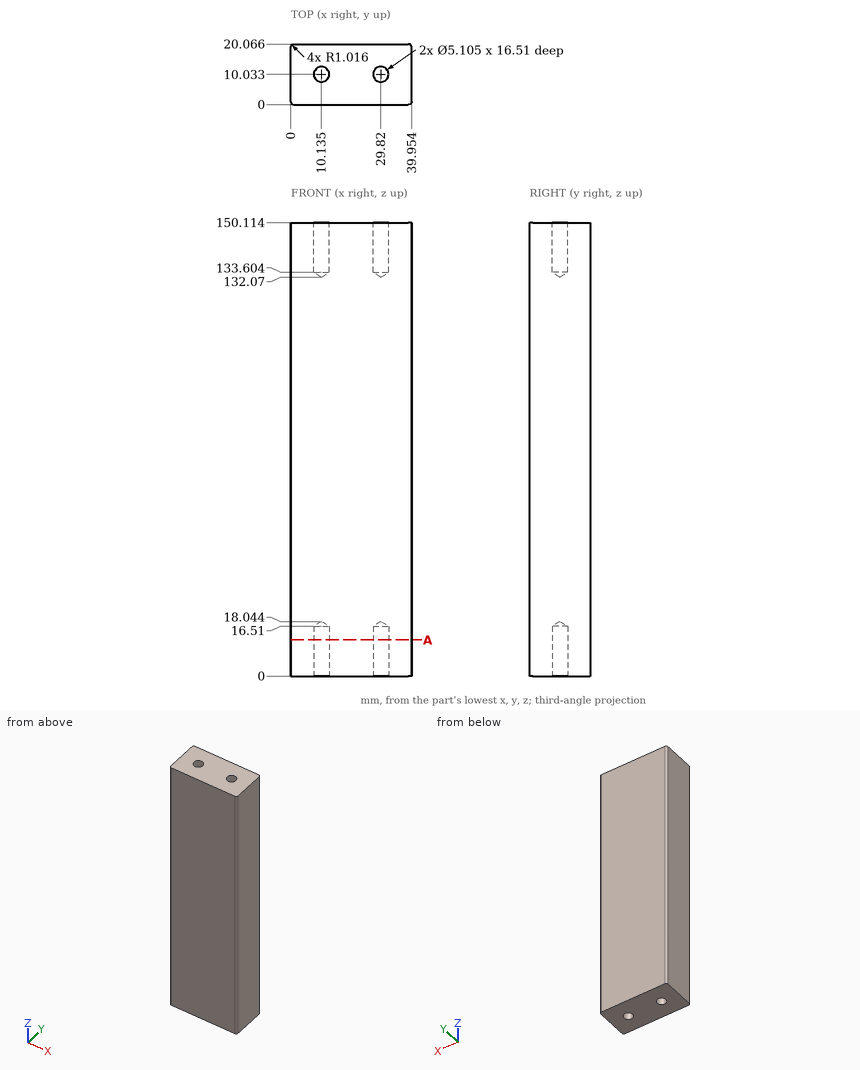
Could you check a few things on this drawing? It's one solid part, dimensions in mm from its lowest x, y, z. Give positions to 0.01 mm unless a question says otherwise; leave off trailing zeros. One line per item, written item: value. Start each with the question number.
1. For P1, Ø8, axis at x = 10.13, y = 10.03, coming from the -Z side; P2, Ø4.5, axis at x = 29.82, y = 10.03, coming from the +Z side (1 decimal); P3, Ø4.5, axis at x = 29.82, y = 10.03, coming from the -Z side, each with a flat end and sliding along its axis, tell me the tip position at first contact or that it passes through.
2. Imagine slicing it at A-A on z = 12. Give the number of separate pieces and of enclosed holes in the cut face, plus the area to 3 significant figures.
3. If I drill on probe 1 along Z at (x, y) = (31, 11), over which ranges is the centre line in solid material (lowest first)?
Values:
1. P1: z = 0
1. P2: z = 133.4
1. P3: z = 16.69
2. separate pieces: 1
2. enclosed holes: 2
2. area: 760 mm²
3. probe 1: 17.13 to 132.99
